from build123d import *

# Parameters (mm, degrees)
SKETCH1_W           = 70
SKETCH1_H           = 70
BOSS_EXTRUDE1_DEPTH = 20
SKETCH2_W           = 70
SKETCH2_H           = 50
CUT_EXTRUDE1_DEPTH  = 10
SKETCH3_R           = 6.85602035
CUT_EXTRUDE2_DEPTH  = 10


with BuildPart() as part:
    # Sketch1 → Boss-Extrude1 (new body)
    with BuildSketch(Plane.XY):
        with Locations((35, 35)):
            Rectangle(SKETCH1_W, SKETCH1_H)
    extrude(amount=BOSS_EXTRUDE1_DEPTH)

    # Sketch2 → Cut-Extrude1 (cut)
    with BuildSketch(Plane.XY.offset(20)):
        with Locations((35, 35)):
            Rectangle(SKETCH2_W, SKETCH2_H)
    extrude(amount=-CUT_EXTRUDE1_DEPTH, mode=Mode.SUBTRACT)

    # Sketch3 → Cut-Extrude2 (cut)
    with BuildSketch(Plane.XY.offset(10)):
        with Locations((35, 35)):
            Circle(SKETCH3_R)
    extrude(amount=-CUT_EXTRUDE2_DEPTH, mode=Mode.SUBTRACT)


solid = part.part
Geometry: final body of the model. Coordinates: model frame, mm. A direction names the side the tool comes from. Round coordinates to 2 decimals unless told otherwise and drop trailing zeros. Write each loop counter-clockwise with the first axis right and the second up, starting at its lowest first coordinate (ties: lowest second). Pieces come first, ordered by that corner, then holes. Notation, with made-up numbers: M 53,-35 L 90,-35 A4 ccw 90,-29 Z; hole C 47,60.5 d4. An arc over 180 degrees is marked long. Write item = value, one per line.
Item 1: Material intervals for line 1 along Y through (x, z) = (35, 7.5); line 2 along Y through (x, z) = (60, 12); line 3 along Z through (x, y) = (67.5, 54.5), sorted ascending. Write a range as [from, to].
Findings:
line_1 = [0, 28.14], [41.86, 70]
line_2 = [0, 10], [60, 70]
line_3 = [0, 10]
Item 2: Pin query (flat end, axial travel): P1, Ø2, axis at x = 49.5, z = 7.5, coming from the -Y side; P2, Ø12.5, axis at x = 35, y = 35, coming from the -Z side; P3, Ø2, axis at x = 53, y = 22.5, coming from the +Z side. Return the tip coordinate at first contact, or that it passes through.
Findings:
P1 = 0
P2 = through
P3 = 10
Item 3: Pull-direction query (X, two-part tool) for faces 1 (the face through (70, 35, 8)), 2 (the face through (42.3, 35.4, 10)), 3 (the face through (0, 35, 8)), 4 (the face through (29.947, 39.634, 5.07)); classes: pulls with the +X half, pulls with the -X half, needs draft (parallel to the pull), parting line crosses it, or undercut.
Findings:
face_1 = pulls with the +X half
face_2 = needs draft
face_3 = pulls with the -X half
face_4 = undercut
Item 4: Section query A-A on x = 35. Return loops of the section in (y, z).
Findings:
outline = M 0,0 L 28.14,0 L 28.14,10 L 10,10 L 10,20 L 0,20 Z; M 41.86,0 L 70,0 L 70,20 L 60,20 L 60,10 L 41.86,10 Z
Item 5: Section query B-B on y = 35. Return loops of the section in (x, z).
Findings:
outline = M 0,0 L 28.14,0 L 28.14,10 L 0,10 Z; M 41.86,0 L 70,0 L 70,10 L 41.86,10 Z
Item 6: Section query D-D on x = 11. Return loops of the section in (y, z), then the cut area to 3 significant figures.
Findings:
outline = M 0,0 L 70,0 L 70,20 L 60,20 L 60,10 L 10,10 L 10,20 L 0,20 Z
area = 900 mm^2
Item 7: Access query for faces 5 (the face through (35, 60, 15)), 6 (the face through (35, 0, 10)). Directions: +Z, -Z, +X, -X, +Y, -Y. A direction counts if a zero-diameter tool reaches every point of the face in a straight line with its end or side. Return the directions, or none.
Findings:
face_5 = +Z, +X, -X
face_6 = +Z, -Z, +X, -X, -Y
Item 8: Section query C-C on z = 3.25. Return loops of the section in (x, y), then the cut area to 3 significant figures.
Findings:
outline = M 0,0 L 70,0 L 70,70 L 0,70 Z; hole C 35,35 d13.71
area = 4,750 mm^2
